Autodesk Inventor part; units mm, degrees
ref_plane "YZ Plane" through (0, 0, 0) normal (1, 0, 0) x (0, 1, 0)
ref_plane "XZ Plane" through (0, 0, 0) normal (0, 1, 0) x (-1, 0, 0)
ref_plane "XY Plane" through (0, 0, 0) normal (0, 0, 1) x (1, 0, 0)
sketch "Sketch2" plane through (0, 0, 0) normal (0, 0, 1) x (1, 0, 0)
  line L0 (-450, -175) -> (450, -175)
  line L1 (450, -175) -> (450, 175)
  line L2 (450, 175) -> (-450, 175)
  line L3 (-450, 175) -> (-450, -175)
  line L4 (-450, -175) -> (450, 175) construction
  line L5 (450, -175) -> (-450, 175) construction
  point P0 (0, 0)
  dimension "d0" = 900
  dimension "d1" = 350
extrude "Plate1" add sketch "Sketch2" along normal mid plane 3.048
sketch "Sketch3" plane through (450, 171.952, 1.524) normal (0, 1, 0) x (-1, 0, 0)
  line L0 (900, 0) -> (0, 0)
  line L1 (0, 0) -> (0, -25)
  line L2 (0, -25) -> (900, -25)
  line L3 (900, -25) -> (900, 0)
edge flange "Flange1" height 25 angle 90 thickness 3.048 bend radius 3.048 thickness toward (0, 1, 0) relief tear relief width 3.048 relief depth 1.524 corner gap 3.048 corner form 2 edges at (0, 175, -1.524) (-450, 0, -1.524) (0, -175, -1.524) (450, 0, -1.524) wall of the first edge with corners at (-450, 171.952, 1.524) (450, 171.952, 1.524) (450, 171.952, -23.476) (-450, 171.952, -23.476)
bend "Bend1"
corner "Corner1"
equation "\"d2\" = Thickness"
equation "\"d3\" = BendReliefWidth"
equation "\"d4\" = BendReliefDepth"
equation "\"d5\" = MinimumRemnant"
equation "\"d6\" = TransitionRadius"
equation "\"d9\" = BendRadius"
equation "\"d10\" = CornerReliefSize"
equation "\"d11\" = GapSize"
equation "\"d12\" = JacobiRadiusSize"
equation "\"BendRadius\" = Thickness"
equation "\"BendReliefWidth\" = Thickness"
equation "\"BendReliefDepth\" = 0.5 * Thickness"
equation "\"CornerReliefSize\" = 4 * Thickness"
equation "\"MinimumRemnant\" = 2 * Thickness"
equation "\"TransitionRadius\" = BendRadius"
equation "\"JacobiRadiusSize\" = BendRadius"
equation "\"GapSize\" = Thickness"
equation "\"Space5\" = 0"
equation "\"Space6\" = 0"
equation "\"Space7\" = 0"
properties part number "TapaDown"
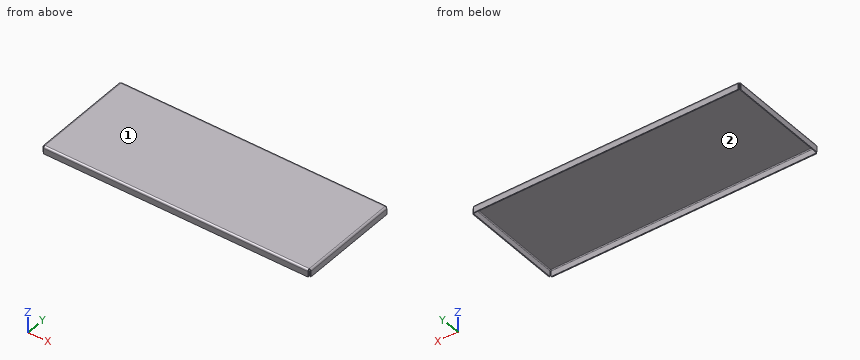
The listing builds one solid part. Answer for the finished solid, in the listing's coordinates (mm). Face numbers are marked on the shaded views. Round coordinates to 2 decimals unless told otherwise and drop trailing zeros. Loops run counter-clockwise (first coordinate to the right, second up) from the corner with the lowest first, then second, coordinate; pieces in that order, holes last. Notation, with made-up numbers: (11.5, 55.5) - (65.5, 55.5) arc R17 cw to (65.5, 66.5) - close; hole circle Ø10 at (-30.75, 15). An arc over 180 degrees is marked (long way). Return JSON: item names as keys, results as strings. Group by question number.
1. The mould has two halves that part along Y. Classify the marked faces 1 and 2: pulls with the +Y half, pulls with the -Y half, needs draft (parallel to the pull), parting line crosses it, or undercut.
2. The part is cut by section A-A on z = -11. Determine the outline of the cut face in (x, y).
3. The part is cut by section B-B on y = -78.5. Determine the outline of the cut face in (x, z).
4. The part is cut by section C-C on x = -368. Determine the outline of the cut face in (y, z).
5. Consider probe 1 along Y at (x, z) = (-247, -6.5); probe 2 along X at (y, z) = (101.5, -18); probe 3 along Z at (x, y) = (-251.5, 76). Determine where each line is inside the solid, lowest interval first.
6. Each of these flat-tipped pins is pushed along its axis until it touches: P1, Ø3, axis at y = -172.5, z = -0.5, coming from the -X side; P2, Ø1, axis at x = 43.5, y = 131.5, coming from the -Z side; P3, Ø5, axis at x = 446.5, z = -2.5, coming from the -Y side; P4, Ø1.5, axis at x = -310.5, z = -4, coming from the +Y side. Where does it stop, or does it pass through?
Resolved:
{
 "1": {"face 1": "needs draft", "face 2": "undercut"},
 "2": {"outline": "(-450, -169.8) - (-446.95, -169.8) - (-446.95, 169.8) - (-450, 169.8) - close; (-444.8, -175) - (444.8, -175) - (444.8, -171.95) - (-444.8, -171.95) - close; (-444.8, 171.95) - (444.8, 171.95) - (444.8, 175) - (-444.8, 175) - close; (446.95, -169.8) - (450, -169.8) - (450, 169.8) - (446.95, 169.8) - close"},
 "3": {"outline": "(-450, -23.48) - (-446.95, -23.48) - (-446.95, -4.57) arc R3.05 cw to (-443.9, -1.52) - (443.9, -1.52) arc R3.05 cw to (446.95, -4.57) - (446.95, -23.48) - (450, -23.48) - (450, -4.57) arc R6.1 ccw to (443.9, 1.52) - (-443.9, 1.52) arc R6.1 ccw to (-450, -4.57) - close"},
 "4": {"outline": "(-175, -23.48) - (-171.95, -23.48) - (-171.95, -4.57) arc R3.05 cw to (-168.9, -1.52) - (168.9, -1.52) arc R3.05 cw to (171.95, -4.57) - (171.95, -23.48) - (175, -23.48) - (175, -4.57) arc R6.1 ccw to (168.9, 1.52) - (-168.9, 1.52) arc R6.1 ccw to (-175, -4.57) - close"},
 "5": {"probe 1": "y = -175 to -171.95, 171.95 to 175", "probe 2": "x = -450 to -446.95, 446.95 to 450", "probe 3": "z = -1.52 to 1.52"},
 "6": {"P1": "stops at x = -443.9", "P2": "stops at z = -1.52", "P3": "stops at y = -169.8", "P4": "stops at y = 175"}
}
